Print and shaded views of the part. All mm, measured from the part's lowest x, y and z. A direction names the side the tool comes from. Coordinates: 2 decimals unless noted, no trailing zeros. Order: outer loops, then holes, each group sorted by start corner. A loop starts at its lowest first (then second) coordinate and runs counter-clockwise, first axis right, second up. Notation, with made-up numbers: (28, 42) - (82, 42) arc R21 ccw to (82, 76) - close; hole circle Ø5 at (-11, 58). An arc over 180 degrees is marked (long way). Write each question's results on one line, items separated by ' | '.
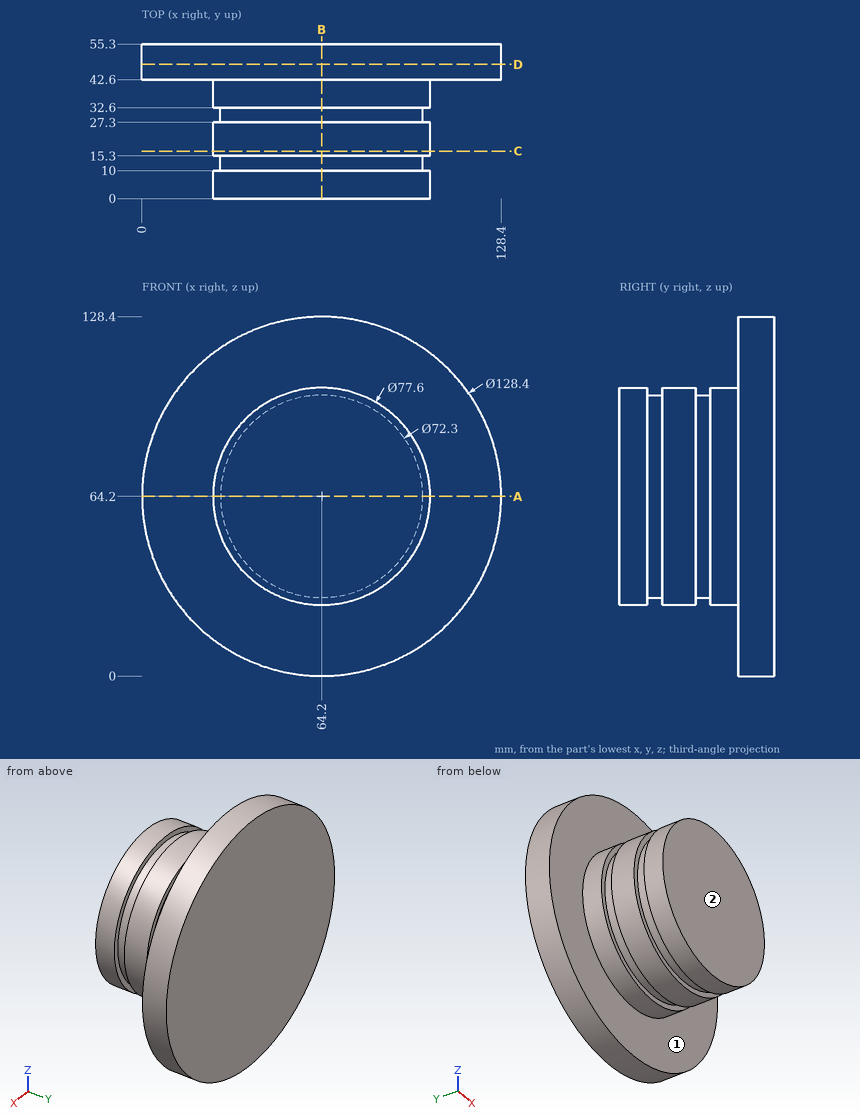
1. Tool access for the marked faces 1 and 2: list every direction of +Z, -Z, +X, -X, +Y, -Y with a clear straight run to the whole face (end or side of a thin tool).
Solved:
face 1: -Y | face 2: +Z, -Z, +X, -X, -Y
2. Probe line 1 (Y direction, x = 32, z = 44); line 2 (Y direction, x = 79.5, z = 5); line 3 (Z direction, x = 65.5, y = 24.5). List the from-to ranges inside material, lowest first.
Solved:
line 1: y = 0 to 10, 15.3 to 27.3, 32.6 to 55.3 | line 2: y = 42.6 to 55.3 | line 3: z = 25.42 to 102.98
3. Band-saw the part on B-B on x = 64.2. Give the cut face in (y, z).
Solved:
outline: (0, 25.4) - (10, 25.4) - (10, 28.05) - (15.3, 28.05) - (15.3, 25.4) - (27.3, 25.4) - (27.3, 28.05) - (32.6, 28.05) - (32.6, 25.4) - (42.6, 25.4) - (42.6, 0) - (55.3, 0) - (55.3, 128.4) - (42.6, 128.4) - (42.6, 103) - (32.6, 103) - (32.6, 100.35) - (27.3, 100.35) - (27.3, 103) - (15.3, 103) - (15.3, 100.35) - (10, 100.35) - (10, 103) - (0, 103) - close
4. Band-saw the part on A-A on z = 64.2. Give the cut face in (x, y), then the cut area to 3 significant figures.
Solved:
outline: (0, 42.6) - (25.4, 42.6) - (25.4, 32.6) - (28.05, 32.6) - (28.05, 27.3) - (25.4, 27.3) - (25.4, 15.3) - (28.05, 15.3) - (28.05, 10) - (25.4, 10) - (25.4, 0) - (103, 0) - (103, 10) - (100.35, 10) - (100.35, 15.3) - (103, 15.3) - (103, 27.3) - (100.35, 27.3) - (100.35, 32.6) - (103, 32.6) - (103, 42.6) - (128.4, 42.6) - (128.4, 55.3) - (0, 55.3) - close | area: 4,880 mm2
5. Band-saw the part on C-C on y = 17. Give the cut face in (x, z), then the cut area to 3 significant figures.
Solved:
outline: circle Ø77.6 at (64.2, 64.2) | area: 4,730 mm2
6. Band-saw the part on D-D on y = 48. Give the cut face in (x, z), then the cut area to 3 significant figures.
Solved:
outline: circle Ø128.4 at (64.2, 64.2) | area: 12,900 mm2
7. Drop flat-ended pins along their axis: pin 1 Ø1 at (x, y) = (89, 34.5) entering from +Z; pin 2 Ø1 at (y, z) = (17, 75) entering from -X; pin 3 Ø1 at (x, y) = (33, 42.5) entering from -Z; pin 4 Ø4 at (x, z) = (20, 114) entering from -Y. Give the stop position or say it passes through.
Solved:
pin 1: stops at z = 94.45 | pin 2: stops at x = 26.79 | pin 3: stops at z = 7.82 | pin 4: passes through
